from build123d import *

# Parameters (mm, degrees)
EXTRUDE_THIN1_DEPTH = 304.8
FILLET1_R           = 1.016


with BuildPart() as part:
    # Sketch1 → Extrude-Thin1 (new body)
    with BuildSketch(Plane.XY):
        with BuildLine():
            Line((0, 0), (-10.31875, 0))
            Line((-10.31875, 0), (-10.31875, 12.199518022))
            Line((-10.31875, 12.199518022), (-7.726000141, 12.199518022))
            Line((-7.726000141, 12.199518022), (-7.726000141, 13.878836266))
            ThreePointArc((-7.726000141, 13.878836266), (-9.572182479, 15.568472968), (-9.26085893, 18.051684409))
            Line((-9.26085893, 18.051684409), (-4.088758773, 25.580941853))
            ThreePointArc((-4.088758773, 25.580941853), (-3.258106429, 27.807165094), (-3.571875, 30.1625))
            Line((-3.571875, 30.1625), (0, 30.1625))
            Line((0, 30.1625), (0, 29.1465))
            Line((0, 29.1465), (-2.264128397, 29.1465))
            ThreePointArc((-2.264128397, 29.1465), (-2.372545269, 26.984258971), (-3.251310814, 25.005670685))
            Line((-3.251310814, 25.005670685), (-8.423410971, 17.476413241))
            ThreePointArc((-8.423410971, 17.476413241), (-8.449647278, 15.58096036), (-6.710000141, 14.827927951))
            Line((-6.710000141, 14.827927951), (-6.710000141, 11.183518022))
            Line((-6.710000141, 11.183518022), (-9.30275, 11.183518022))
            Line((-9.30275, 11.183518022), (-9.30275, 1.016))
            Line((-9.30275, 1.016), (0, 1.016))
            Line((0, 1.016), (0, 0))
        make_face()
    extrude(amount=-EXTRUDE_THIN1_DEPTH)

    # Fillet1
    fillet1_edges = [part.edges().sort_by_distance(p)[0] for p in [
        (-10.31875, 0, -152.4),
        (-10.31875, 12.199518022, -152.4),
        (-3.571875, 30.1625, -152.4),
        (-6.710000141, 14.827927951, -152.4),
        (-6.710000141, 11.183518022, -152.4),
    ]]
    fillet(fillet1_edges, radius=FILLET1_R)


solid = part.part
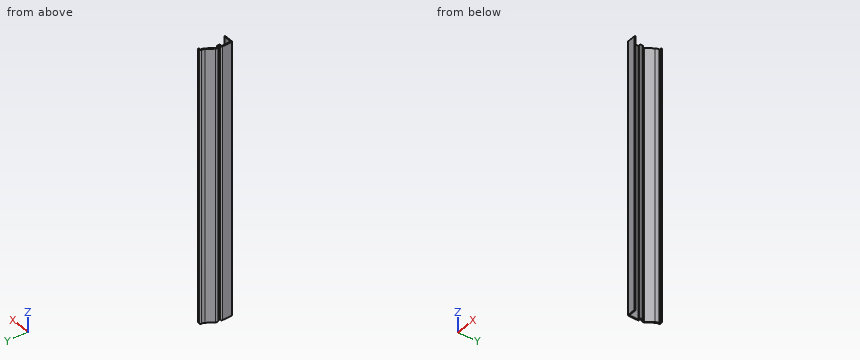
The listing builds one solid part. Answer for the finished solid, in the listing's coordinates (mm). Coordinates: 2 decimals unless noted, no trailing zeros. Order: outer loops, then holes, each group sorted by start corner. A loop starts at its lowest first (then second) coordinate and runs counter-clockwise, first axis right, second up. Notation, with made-up numbers: (42.25, 48) -> (93.25, 48) arc R14 cw to (93.25, 65) -> close; hole circle Ø9 at (-37, 24). An arc over 180 degrees is marked (long way). Answer in a Markdown table with one row per item. Add a question column.
Item 1: Find section A-A (z = -277.5). Write down the section's boundary in (x, y), then the cut area to 3 significant figures.
Item 2: Find section B-B (y = 7.5). Write down the section's boundary in (x, z), then the cut area to 3 significant figures.
Item 3: Find the intervals of material crossed by L1, parallel to Y at x = -1.25, z = -260.5; L2, parallel to Y at x = -7, z = -236.5; L3, parallel to Y at x = -8.25, z = -51, in increasing order. Write a range as from..to.
Item 4: Each of these flat-tipped pins is pushed along its axis until it touches: P1, Ø1.3, axis at y = 12.5, z = -95, coming from the +X side; P2, Ø3, axis at x = -6, z = -223, coming from the +Y side; P3, Ø0.8, axis at x = -8, z = -85.5, coming from the +Y side. Where does it stop, or does it pass through?
Result set:
| question | item | result |
|---|---|---|
| 1 | outline | (-10.32, 1.02) arc R1.02 ccw to (-9.3, 0) -> (0, 0) -> (0, 1.02) -> (-9.3, 1.02) -> (-9.3, 11.18) -> (-7.73, 11.18) arc R1.02 ccw to (-6.71, 12.2) -> (-6.71, 13.88) arc R1.02 ccw to (-7.46, 14.86) arc R1.71 cw to (-8.42, 17.48) -> (-3.25, 25.01) arc R5.92 ccw to (-2.26, 29.15) -> (0, 29.15) -> (0, 30.16) -> (-2.26, 30.16) arc R1.02 ccw to (-3.27, 29.01) arc R4.9 cw to (-4.09, 25.58) -> (-9.26, 18.05) arc R2.72 ccw to (-7.73, 13.88) -> (-7.73, 12.2) -> (-9.3, 12.2) arc R1.02 ccw to (-10.32, 11.18) -> close |
| 1 | area | 47.0 mm² |
| 2 | outline | (-10.32, -304.8) -> (-9.3, -304.8) -> (-9.3, 0) -> (-10.32, 0) -> close |
| 2 | area | 310 mm² |
| 3 | L1 | y = 0..1.02, 29.15..30.16 |
| 3 | L2 | y = 0..1.02, 11.49..14.59, 19.55..21.34 |
| 3 | L3 | y = 0..1.02, 11.18..12.2, 14.08..15.33, 17.73..19.52 |
| 4 | P1 | stops at x = -6.71 |
| 4 | P2 | stops at y = 24.98 |
| 4 | P3 | stops at y = 20.47 |
